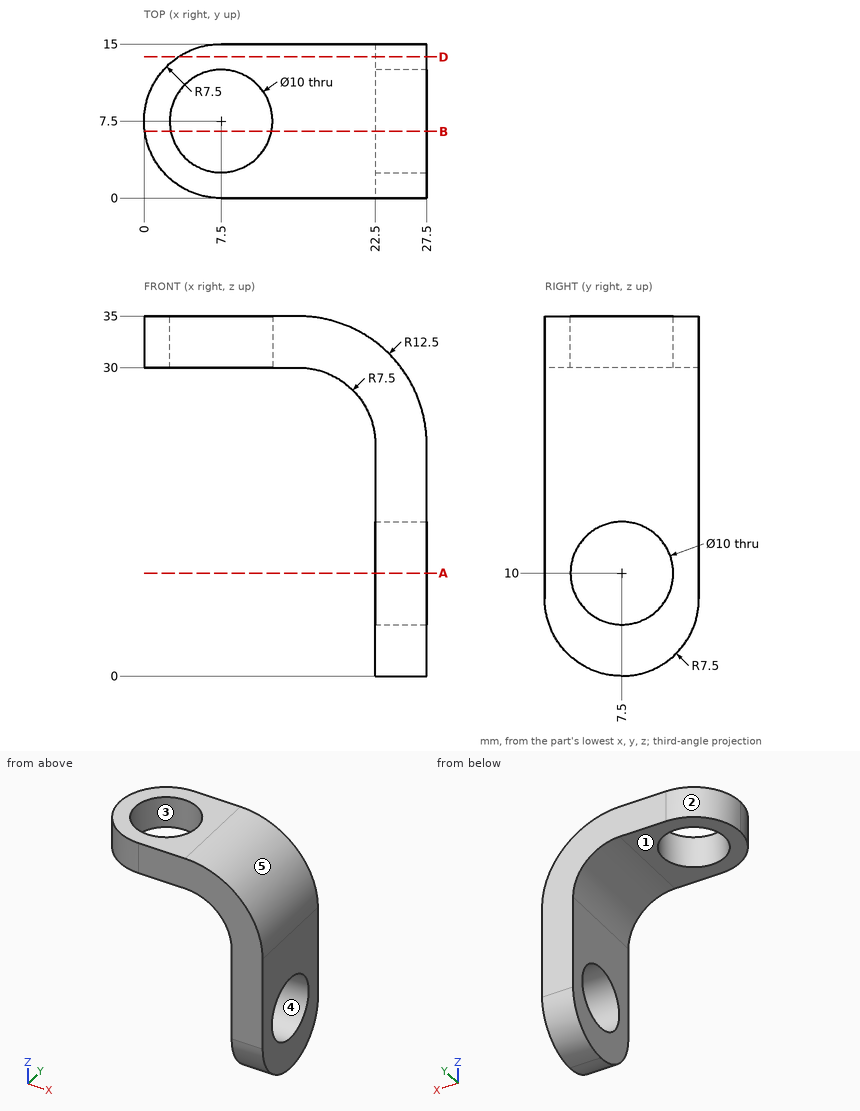
Source: three-view drawing plus pictorial views. Frame: mm from the lowest corner of the part. A direction names the side the tool comes from. Give positions to 0.01 mm unless a question says otherwise; leave off trailing zeros. Loops run counter-clockwise (first coordinate to the right, second up) from the corner with the lowest first, then second, coordinate; pieces in that order, holes last. Notation, with made-up numbers: (35.25, 84) -> (75.25, 84) arc R15 cw to (75.25, 99) -> close; hole circle Ø2 at (-12, 56). An arc over 180 degrees is marked (long way). Put each result on its own line as item: value. Start each with the question number.
1) Cut plane B-B (y = 6.5). Return loops of the section in (x, z).
2) Material intervals for probe 1 along Y at (x, z) = (7.5, 32.55); probe 2 along X at (y, z) = (12.5, 15); probe 3 along X at (y, z) = (8.5, 31), sorted ascending.
3) Draft query along X for the marked faces 3, 4 and 5. Return one class per face: released by +X, released by -X, zero draft, split by the parting line, or undercut.
4) Contact query for flat-ended pins moving along their axis: P1, Ø2, axis at x = 21, z = 16.5, coming from the -Y side (3 decimals); P2, Ø4.5, axis at x = 5.5, y = 10, coming from the -Z side; P3, Ø2, axis at y = 8.5, z = 15, coming from the -X side. Output: stop coordinate, or through.
5) Cut plane D-D (y = 13.75). Return loops of the section in (x, z), then the cut area to 4 significant figures.
6) Cut plane A-A (z = 10). Return loops of the section in (x, y), then the cut area to 3 significant figures.
7) Reachability of the marked faces 1 and 2 from +Z, -Z, +X, -X, +Y, -Y: full face, straight path, thin tool, end or side. Return the list, or none.
Results are:
1. outline: (0.07, 30) -> (2.6, 30) -> (2.6, 35) -> (0.07, 35) -> close; (12.4, 30) -> (15, 30) arc R7.5 cw to (22.5, 22.5) -> (22.5, 14.9) -> (27.5, 14.9) -> (27.5, 22.5) arc R12.5 ccw to (15, 35) -> (12.4, 35) -> close; (22.5, 0.07) -> (27.5, 0.07) -> (27.5, 5.1) -> (22.5, 5.1) -> close
2. probe 1: y = 0 to 2.5, 12.5 to 15
2. probe 2: x = 22.5 to 27.5
2. probe 3: x = 0.07 to 2.6, 12.4 to 24.17
3. face 3: undercut
3. face 4: zero draft
3. face 5: released by +X
4. P1: passes through
4. P2: stops at z = 30
4. P3: stops at x = 22.5
5. outline: (3.35, 30) -> (15, 30) arc R7.5 cw to (22.5, 22.5) -> (22.5, 3.35) -> (27.5, 3.35) -> (27.5, 22.5) arc R12.5 ccw to (15, 35) -> (3.35, 35) -> close
5. area: 232.5 mm2
6. outline: (22.5, 0) -> (27.5, 0) -> (27.5, 2.5) -> (22.5, 2.5) -> close; (22.5, 12.5) -> (27.5, 12.5) -> (27.5, 15) -> (22.5, 15) -> close
6. area: 25.0 mm2
7. face 1: -Z, -X, +Y, -Y
7. face 2: +Z, -Z, -X, +Y
